Part model, mm, in its own coordinate system. Face numbers are marked on the shaded views. A direction names the side the tool comes from. Coordinates: 2 decimals unless noted, no trailing zeros. Write each loop counter-clockwise with the first axis right and the second up, starting at its lowest first coordinate (ties: lowest second). Pieces come first, ordered by that corner, then holes. Notation, with made-up numbers: (-36.5, 6) - (7.5, 6) arc R26 ccw to (7.5, 44) - close; hole circle Ø2 at (63, 86). An arc over 180 degrees is marked (long way). Write each question's results on one line, items separated by ' | '.
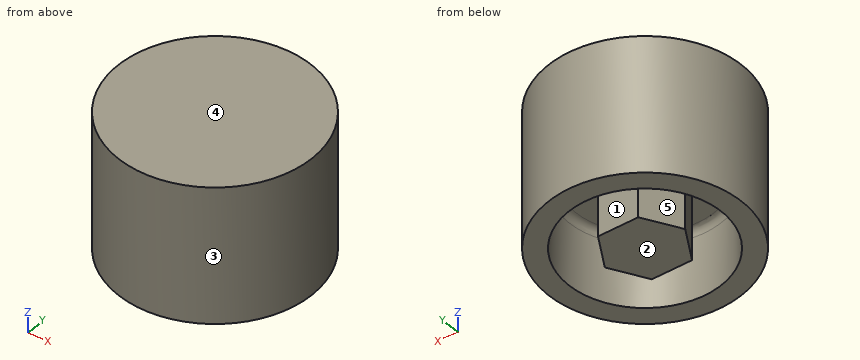
from build123d import *

# Parameters (mm, degrees)
CYLINDER_R        = 2.8
CYLINDER_DEPTH    = 2.54
POCKET_DEPTH      = 5
FILLET_R          = 0.25
CYLINDER001_R     = 3.55
CYLINDER001_DEPTH = 5


with BuildPart() as bolt:
    # Cylinder → Cylinder (new body)
    with BuildSketch(Plane.XY):
        Circle(CYLINDER_R)
    extrude(amount=CYLINDER_DEPTH)

    # Sketch → Pocket (cut)
    with BuildSketch(Plane.XY.offset(2.54)):
        Polygon((-0.733235, 1.27), (-1.46647, 0), (-0.733235, -1.27), (0.733235, -1.27), (1.46647, 0), (0.733235, 1.27), align=None)
    extrude(amount=-POCKET_DEPTH, mode=Mode.SUBTRACT)

    # Fillet
    fillet_edges = [bolt.edges().sort_by_distance(p)[0] for p in [
        (-2.8, 0, 2.54),
    ]]
    fillet(fillet_edges, radius=FILLET_R)


with BuildPart() as bolt_hook:
    # Cylinder001 → Cylinder001 (new body)
    with BuildSketch(Plane.XY):
        Circle(CYLINDER001_R)
    extrude(amount=CYLINDER001_DEPTH)

    # Cut: cut Bolt
    add(bolt.part, mode=Mode.SUBTRACT)


solid = bolt_hook.part
(1) 3-axis set-ups, long thin cutter, end or side, ignore diameter. For the marked faces 1 and 2: which of +Z, -Z, +X, -X, +Y, -Y reach the whole face in a straight line?
Return value:
face 1: -Z | face 2: -Z, +X, -X, +Y, -Y
(2) Saw through at C-C on z = 3.95. Write the cut outline in (x, y).
Return value:
outline: circle Ø7.1 at (0, 0)
(3) Saw through at A-A on z = 1.2. Write the cut outline in (x, y), then the cut area to 3 significant figures.
Return value:
outline: circle Ø7.1 at (0, 0); (-1.47, 0) - (-0.73, -1.27) - (0.73, -1.27) - (1.47, 0) - (0.73, 1.27) - (-0.73, 1.27) - close; hole circle Ø5.6 at (0, 0) | area: 20.5 mm^2
(4) Two-plate mould, pull along X, no slides. Class the marked faces 3, 4 and 5: released by +X, released by -X, zero draft, split by the parting line, or undercut.
Return value:
face 3: split by the parting line | face 4: zero draft | face 5: undercut
(5) Saw through at D-D on x = -3. Write the cut outline in (y, z), then the cut area to 3 significant figures.
Return value:
outline: (-1.9, 0) - (1.9, 0) - (1.9, 5) - (-1.9, 5) - close | area: 19.0 mm^2
(6) Flat gauge pins, fed straight in: P1, Ø2, axis at y = -0.5, z = 2.5, coming from the +X side; P2, Ø2, axis at x = -2, z = 2.5, coming from the -Y side. Where does each tip first touch, or does it go through?
Return value:
P1: stops at x = 3.55 | P2: stops at y = -3.41
(7) Wall check: line 1 (Y direction, x = 0, z = 1.6); line 2 (Y direction, x = 1, z = 2.05); line 3 (X direction, y = -0.5, z = 1.6) (3 decimals). Give the ranges that are in metal, low to high. Write a range as from..to.
Return value:
line 1: y = -3.55..-2.8, -1.27..1.27, 2.8..3.55 | line 2: y = -3.41..-2.62, -0.81..0.81, 2.62..3.41 | line 3: x = -3.515..-2.755, -1.178..1.178, 2.755..3.515
(8) Saw through at B-B on x = 0. Write the cut outline in (y, z).
Return value:
outline: (-3.55, 0) - (-2.8, 0) - (-2.8, 2.29) arc R0.25 cw to (-2.55, 2.54) - (-1.27, 2.54) - (-1.27, 0) - (1.27, 0) - (1.27, 2.54) - (2.55, 2.54) arc R0.25 cw to (2.8, 2.29) - (2.8, 0) - (3.55, 0) - (3.55, 5) - (-3.55, 5) - close
